The listing builds one solid part. Answer for the finished solid, in the listing's coordinates (mm). A direction names the side the tool comes from. Give positions to 0.01 mm unless a question says otherwise; leave off trailing zeros. Order: outer loops, then holes, each group sorted by start corner. A loop starts at its lowest first (then second) coordinate and runs counter-clockwise, first axis right, second up. Notation, with made-up numbers: M -39.75,-11 L -19.75,-11 A30 cw -19.75,20 Z; hole C -4.75,69.25 d6. An arc over 180 degrees is marked long. Answer as a JSON object with one key per item and string values. Group by question number.
```python
from build123d import *

# Parameters (mm, degrees)
SKETCH1_R           = 7.5
BOSS_EXTRUDE1_DEPTH = 15
SKETCH7_R           = 2.5
CUT_EXTRUDE2_DEPTH  = 5
SKETCH2_R           = 15
BOSS_EXTRUDE2_DEPTH = 100
CUT_EXTRUDE3_DEPTH  = 52
SKETCH9_R           = 15
BOSS_EXTRUDE4_DEPTH = 52
SKETCH10_R          = 2.5
CUT_EXTRUDE4_DEPTH  = 5


with BuildPart() as part:
    # Sketch1 → Boss-Extrude1 (new body)
    with BuildSketch(Plane.XY):
        Circle(SKETCH1_R)
    extrude(amount=-BOSS_EXTRUDE1_DEPTH)

    # Sketch7 → Cut-Extrude2 (cut)
    with BuildSketch(Plane.XY):
        Circle(SKETCH7_R)
    extrude(amount=-CUT_EXTRUDE2_DEPTH, mode=Mode.SUBTRACT)

    # Sketch2 → Boss-Extrude2 (add)
    with BuildSketch(Plane(origin=(0, 0, -15), x_dir=(-1, 0, 0), z_dir=(0, 0, -1))):
        Circle(SKETCH2_R)
    extrude(amount=BOSS_EXTRUDE2_DEPTH)

    # Sketch8 → Cut-Extrude3 (cut, symmetric)
    with BuildSketch(Plane(origin=(0, 0, 0), x_dir=(1, 0, 0), z_dir=(0, 1, 0))):
        with BuildLine():
            Line((15, 165), (-15, 165))
            Line((-15, 165), (-15, 100))
            ThreePointArc((-15, 100), (0, 115), (15, 100))
            Line((15, 100), (15, 165))
        make_face()
    extrude(amount=CUT_EXTRUDE3_DEPTH, both=True, mode=Mode.SUBTRACT)

    # Sketch9 → Boss-Extrude4 (add, symmetric)
    with BuildSketch(Plane(origin=(0, 0, 0), x_dir=(1, 0, 0), z_dir=(0, 1, 0))):
        with Locations(Location((0, 100, 0), (0, 0, 270))):
            Circle(SKETCH9_R)
    extrude(amount=BOSS_EXTRUDE4_DEPTH, both=True)

    # Sketch10 → Cut-Extrude4 (cut)
    with BuildSketch(Plane.XZ.offset(52)):
        with Locations(Location((0, -100, 0), (0, 0, 270))):
            Circle(SKETCH10_R)
    cut_extrude4 = extrude(amount=-CUT_EXTRUDE4_DEPTH, mode=Mode.SUBTRACT)

    # Mirror1: Cut-Extrude4 across plane
    add(cut_extrude4.mirror(Plane.ZX), mode=Mode.SUBTRACT)


solid = part.part
```
Item 1: Determine the mould class of faces 5 (the cylindrical face through (-0.54, -2.44, -2.46)), 6 (the flat face through (0, 47, -100)), 7 (the cylindrical face through (3.252, -14.643, -56.905)), 8 (the flat face through (4, 7, -15)) for opening direction X: released by +X, released by -X, zero draft, split by the parting line, or undercut.
Item 2: Consider probe 1 along X at (y, z) = (-49.7, -100); probe 2 along Z at (x, y) = (0.75, 13.5); probe 3 along Z at (x, y) = (0.75, -45). Determine where each line is inside the solid, lowest interval first. Write a range as from..to.
Item 3: Section B-B (z = -36) is taken. Determine the outline of the cut face in (x, y).
Item 4: Section D-D (z = -105) is taken. Determine the outline of the cut face in (x, y).
Item 5: Section C-C (y = 35.5) is taken. Determine the outline of the cut face in (x, z).
Item 6: Flat-ended cylindrical pins translate along their axes: P1, Ø4.5, axis at x = 0, z = -100, coming from the +Y side; P2, Ø5, axis at x = 6, z = -59.5, coming from the -Y side; P3, Ø3, axis at x = 0, z = -48.5, coming from the +Y side. Find the tip coordinate at first contact, or state that the pin passes through.
Item 7: Section A-A (x = 0) is taken. Determine the outline of the cut face in (y, z).
Item 8: A tool of negligible diameter and unlimited length cuts with its end or side. For faces 1 (the flat face through (0, -47, -100)), 2 (the flat face through (-3, 52, -100)), 3 (the cylindrical face through (0.751, 49.535, -102.385)), 4 (the cylindrical face through (-7.493, 0.33, -7.395)), from which of +Z, -Z, +X, -X, +Y, -Y can it reach the whole face along a straight path? Write none if from no direction.
Values found:
{
 "1": {"face 5": "undercut", "face 6": "undercut", "face 7": "split by the parting line", "face 8": "zero draft"},
 "2": {"probe 1": "x = -15..-2.5, 2.5..15", "probe 2": "z = -114.98..-15", "probe 3": "z = -114.98..-85.02"},
 "3": {"outline": "C 0,0 d30"},
 "4": {"outline": "M -14.14,-52 L 14.14,-52 L 14.14,52 L -14.14,52 Z"},
 "5": {"outline": "C 0,-100 d30"},
 "6": {"P1": "stops at y = 47", "P2": "stops at y = -14.59", "P3": "stops at y = 15"},
 "7": {"outline": "M -52,-115 L 52,-115 L 52,-102.5 L 47,-102.5 L 47,-97.5 L 52,-97.5 L 52,-85 L 15,-85 L 15,-15 L 7.5,-15 L 7.5,0 L 2.5,0 L 2.5,-5 L -2.5,-5 L -2.5,0 L -7.5,0 L -7.5,-15 L -15,-15 L -15,-85 L -52,-85 L -52,-97.5 L -47,-97.5 L -47,-102.5 L -52,-102.5 Z"},
 "8": {"face 1": "-Y", "face 2": "+Z, -Z, +X, -X, +Y", "face 3": "+Y", "face 4": "+Z"}
}
